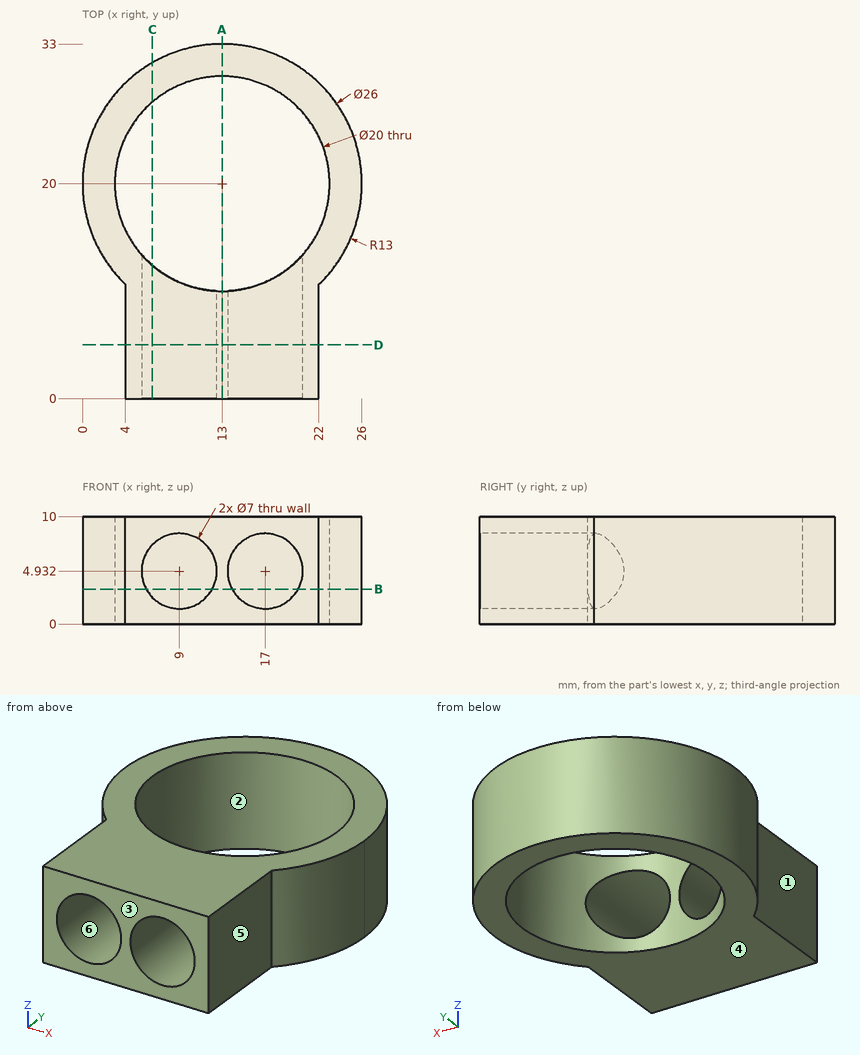
Could you check a few things on this drawing? It's one solid part, dimensions in mm from its lowest x, y, z. A direction names the side the tool comes from. Coordinates: 2 decimals unless noted, no trailing zeros. Order: outer loops, then holes, each group sorted by start corner. A loop starts at its lowest first (then second) coordinate and runs counter-clockwise, first axis right, second up. Notation, with made-up numbers: M 16.5,-9 L 72.5,-9 A14 cw 72.5,-3 Z; hole C -20.75,69.25 d2. An arc over 180 degrees is marked long. Answer as a JSON object with one key per item and string values. Group by question number.
(1) Suppose I cut it at D-D, the plane y = 5. Please give me the cut outline in (x, z).
(2) Suppose I cut it at B-B, the plane z = 3.25. Please give me the cut outline in (x, y).
(3) Suppose I cut it at C-C, the plane x = 6.5. Please give me the cut outline in (y, z).
(4) Suppose I cut it at A-A, the plane x = 13. Please give me the cut outline in (y, z).
(5) If we mould it in two halves opening along Y, with no side actions, what happens to the marked faces 1, 2 and 3? For each: released by +Y, released by -Y, zero draft, split by the parting line, or undercut.
(6) Which directions (+Z, -Z, +X, -X, +Y, -Y) give clear straight access to the entire face, cutting with the end or side of a thin tool? Please do the marked faces 4, 5 and 6.
(7) I need wall thicknesses on probe 1 along Y at (x, z) = (13, 8.25); probe 2 along Z at (x, y) = (9, 4.75); probe 3 along X at (y, z) = (8, 2.25). Which ranges of each line are inside material? Lowest first, please.
(8) For pin 1 (2 mm diameter, centred on y = 10.5, z = 4.5, fed in from -X); pin 2 (5 mm diameter, centred on y = 7.5, z = 5.5, fed in from -X); pin 3 (1.5 mm diameter, centred on y = 29, z = 2.5, fed in from -X), each with a flat end and sliding along its axis, tell me the tip position at first contact or that it passes through.
Values found:
{
 "1": {"outline": "M 4,0 L 22,0 L 22,10 L 4,10 Z; hole C 9,4.93 d7; hole C 17,4.93 d7"},
 "2": {"outline": "M 4,0 L 5.93,0 L 5.93,12.93 A10 cw long 20.07,12.93 L 20.07,0 L 22,0 L 22,10.62 A13 ccw long 4,10.62 Z; M 12.07,0 L 13.93,0 L 13.93,10.04 A10 cw 12.07,10.04 Z"},
 "3": {"outline": "M 0,0 L 12.4,0 L 12.4,2.48 L 0,2.48 Z; M 0,7.38 L 12.4,7.38 L 12.4,10 L 0,10 Z; M 27.6,0 L 31.26,0 L 31.26,10 L 27.6,10 Z"},
 "4": {"outline": "M 0,0 L 10,0 L 10,10 L 0,10 Z; M 30,0 L 33,0 L 33,10 L 30,10 Z"},
 "5": {"face 1": "zero draft", "face 2": "undercut", "face 3": "released by -Y"},
 "6": {"face 4": "-Z, +X, -X, +Y, -Y", "face 5": "+Z, -Z, +X, -Y", "face 6": "-Y"},
 "7": {"probe 1": "y = 0 to 10, 30 to 33", "probe 2": "z = 0 to 1.43, 8.43 to 10", "probe 3": "x = 4 to 6.75, 11.25 to 14.75, 19.25 to 22"},
 "8": {"pin 1": "stops at x = 3.16", "pin 2": "stops at x = 4", "pin 3": "stops at x = 2.95"}
}
